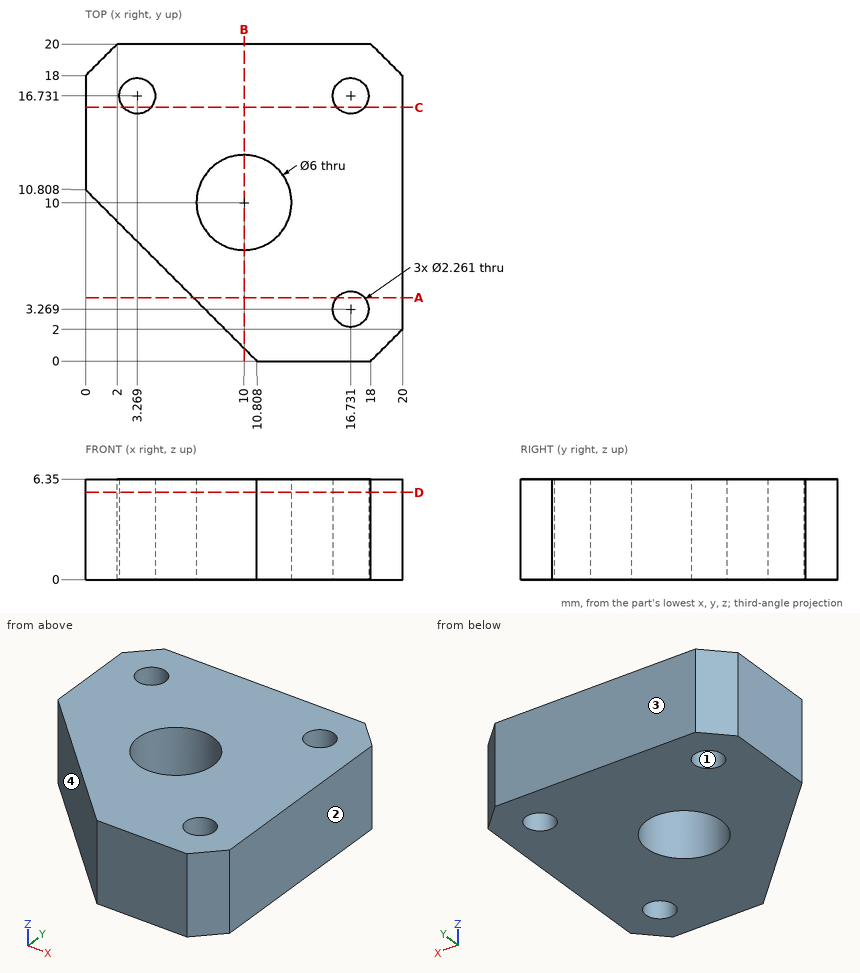
Here's the drawing with two shaded views (mm, measured from the low corner). I have some questions. Give positions to 0.01 mm unless a question says otherwise; leave off trailing zeros. Write each loop counter-clockwise with the first axis right and the second up, starting at its lowest first coordinate (ties: lowest second). Pieces come first, ordered by that corner, then holes. Notation, with made-up numbers: (3.25, 56.5) -> (52.25, 56.5) arc R11 ccw to (52.25, 76.5) -> close; hole circle Ø6 at (2, 89). An arc over 180 degrees is marked (long way). Answer as a JSON object with one key per item and string values. Group by question number.
Item 1: Suppose I cut it at A-A (y = 4). Please give me the cut outline in (x, z).
Item 2: Suppose I cut it at D-D (z = 5.5). Please give me the cut outline in (x, y), plus the area to 3 significant figures.
Item 3: I'm going to push a flat-ended pin straight in: P1, Ø1.5, axis at x = 6, z = 1, coming from the -Y side. Where does the tip first touch, or does it pass through?
Item 4: Suppose I cut it at C-C (y = 16). Please give me the cut outline in (x, z), plus the area to 3 significant figures.
Item 5: Suppose I cut it at B-B (x = 10). Please give me the cut outline in (y, z).
Item 6: We'd pull the mould along Y, two halves only. Please class the marked faces 1, 2, 3 and 4: +Y half, -Y half, draft (parallel to the pull), parting line (faces both ways), or undercut.
Item 7: Please list where these lines run through material, in increasing order: line 1 (Y direction, x = 17, z = 1.75); line 2 (Y direction, x = 17.5, z = 0.75); line 3 (X direction, y = 16, z = 5.5) (1 decimal). Write a range as [from, to].
Findings:
{
 "1": {"outline": "(6.81, 0) -> (15.87, 0) -> (15.87, 6.35) -> (6.81, 6.35) -> close; (17.59, 0) -> (20, 0) -> (20, 6.35) -> (17.59, 6.35) -> close"},
 "2": {"outline": "(0, 10.81) -> (10.81, 0) -> (18, 0) -> (20, 2) -> (20, 18) -> (18, 20) -> (2, 20) -> (0, 18) -> close; hole circle Ø2.26 at (3.27, 16.73); hole circle Ø6 at (10, 10); hole circle Ø2.26 at (16.73, 3.27); hole circle Ø2.26 at (16.73, 16.73)", "area": "295 mm²"},
 "3": {"P1": "stops at y = 4.06"},
 "4": {"outline": "(0, 0) -> (2.41, 0) -> (2.41, 6.35) -> (0, 6.35) -> close; (4.13, 0) -> (15.87, 0) -> (15.87, 6.35) -> (4.13, 6.35) -> close; (17.59, 0) -> (20, 0) -> (20, 6.35) -> (17.59, 6.35) -> close", "area": "105 mm²"},
 "5": {"outline": "(0.81, 0) -> (7, 0) -> (7, 6.35) -> (0.81, 6.35) -> close; (13, 0) -> (20, 0) -> (20, 6.35) -> (13, 6.35) -> close"},
 "6": {"face 1": "undercut", "face 2": "draft", "face 3": "+Y half", "face 4": "-Y half"},
 "7": {"line 1": "y = [0, 2.17], [4.37, 15.63], [17.83, 20]", "line 2": "y = [0, 2.44], [4.1, 15.9], [17.56, 20]", "line 3": "x = [0, 2.4], [4.1, 15.9], [17.6, 20]"}
}
